For this review, use the dimensioned drawing (mm, ordinates from the lowest corner) and the shaded views. Coordinates: 2 decimals unless noted, no trailing zeros. Write each loop counter-clockwise with the first axis right and the second up, starting at its lowest first coordinate (ties: lowest second). Pieces come first, ordered by that corner, then holes. Notation, with made-up numbers: (29, 50) - (52, 50) arc R27 cw to (52, 76) - close; hole circle Ø10 at (89, 87). An arc over 180 degrees is marked (long way). Put each result on its own line as item: value.
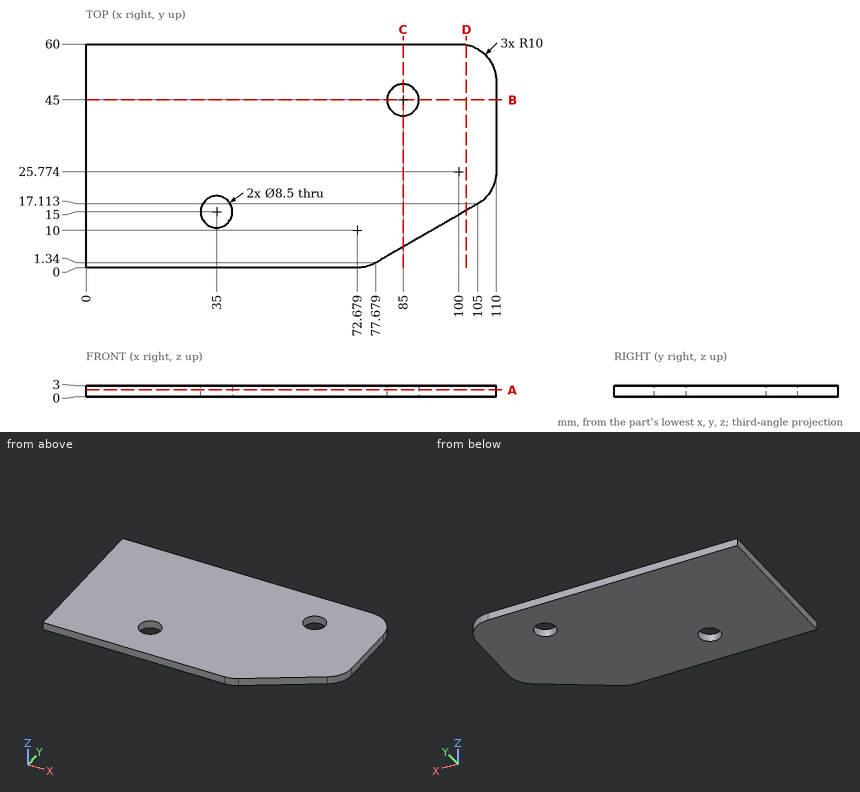
1. Consider section B-B on y = 45. State the section outline as (x, z) points.
Determined:
outline: (0, 0) - (80.75, 0) - (80.75, 3) - (0, 3) - close; (89.25, 0) - (110, 0) - (110, 3) - (89.25, 3) - close
2. Consider section A-A on z = 1.9. State the section outline as (x, y) points, plus the area to 3 significant figures.
Determined:
outline: (0, 0) - (72.68, 0) arc R10 ccw to (77.68, 1.34) - (105, 17.11) arc R10 ccw to (110, 25.77) - (110, 50) arc R10 ccw to (100, 60) - (0, 60) - close; hole circle Ø8.5 at (35, 15); hole circle Ø8.5 at (85, 45)
area: 6,110 mm^2
3. Consider section C-C on x = 85. State the section outline as (y, z) points, plus the area to 3 significant figures.
Determined:
outline: (5.57, 0) - (40.75, 0) - (40.75, 3) - (5.57, 3) - close; (49.25, 0) - (60, 0) - (60, 3) - (49.25, 3) - close
area: 138 mm^2
4. To check wall thickness, follow probe 1 along Y at (x, z) = (35, 0.8); probe 2 along X at (y, z) = (42, 0.7); probe 3 along Y at (x, z) = (31.5, 0.4). State the ranges of each line that lie inside material, in increasing order.
Determined:
probe 1: y = 0 to 10.75, 19.25 to 60
probe 2: x = 0 to 81.99, 88.01 to 110
probe 3: y = 0 to 12.59, 17.41 to 60
5. Consider section D-D on x = 102. State the section outline as (y, z) points, plus the area to 3 significant figures.
Determined:
outline: (15.38, 0) - (59.8, 0) - (59.8, 3) - (15.38, 3) - close
area: 133 mm^2
